from build123d import *

# Parameters (mm, degrees)
SKETCH_1_W          = 117
SKETCH_1_H          = 152
SKETCH_1_R          = 1.525
EXTRUDE_1_DEPTH     = 1
SKETCH_2_R          = 97.5
SKETCH_2_W          = 62.201961009
SKETCH_2_H          = 115
CUT_EXTRUDE_1_DEPTH = 10
SKETCH_3_W          = 20
SKETCH_3_H          = 37.999993186
CUT_EXTRUDE_2_DEPTH = 10
FILLET_1_R          = 2
SKETCH_6_W          = 4
SKETCH_6_H          = 115
EXTRUDE_2_DEPTH     = 1


with BuildPart() as part:
    # 草图1 → 凸台-拉伸1 (new body)
    with BuildSketch(Plane.XY):
        with Locations((38.5, 0)):
            Rectangle(SKETCH_1_W, SKETCH_1_H)
        with Locations((0, 72)):
            Circle(SKETCH_1_R, mode=Mode.SUBTRACT)
        with Locations((0, -72)):
            Circle(SKETCH_1_R, mode=Mode.SUBTRACT)
        with Locations((20, 72)):
            Circle(SKETCH_1_R, mode=Mode.SUBTRACT)
        with Locations((82, 72)):
            Circle(SKETCH_1_R, mode=Mode.SUBTRACT)
        with Locations((82, -72)):
            Circle(SKETCH_1_R, mode=Mode.SUBTRACT)
        with Locations((20, -72)):
            Circle(SKETCH_1_R, mode=Mode.SUBTRACT)
    extrude(amount=EXTRUDE_1_DEPTH)

    # 草图2 → 切除-拉伸1 (cut)
    with BuildSketch(Plane(origin=(0, 0, 0), x_dir=(-1, 0, 0), z_dir=(0, 0, -1))):
        with Locations((101, 0)):
            Circle(SKETCH_2_R)
        with Locations((-65.899019495, 5.300000572)):
            Rectangle(SKETCH_2_W, SKETCH_2_H)
    extrude(amount=-CUT_EXTRUDE_1_DEPTH, mode=Mode.SUBTRACT)

    # 草图3 → 切除-拉伸2 (cut)
    with BuildSketch(Plane(origin=(0, 0, 0), x_dir=(-1, 0, 0), z_dir=(0, 0, -1))):
        with Locations((-30.6, 8.999996593)):
            Rectangle(SKETCH_3_W, SKETCH_3_H)
    extrude(amount=-CUT_EXTRUDE_2_DEPTH, mode=Mode.SUBTRACT)

    # 圆角1
    fillet_1_edges = [part.edges().sort_by_distance(p)[0] for p in [
        (-20, 54.270157545, 0.5),
        (-20, -54.270157545, 0.5),
        (34.798038991, 62.800000572, 0.5),
        (34.798038991, -52.199999428, 0.5),
        (34.798038991, -10, 0.5),
        (34.798038991, 27.999993186, 0.5),
        (20.6, 27.999993186, 0.5),
        (20.6, -10, 0.5),
        (-20, 76, 0.5),
        (97, 76, 0.5),
        (97, -76, 0.5),
        (-20, -76, 0.5),
    ]]
    fillet(fillet_1_edges, radius=FILLET_1_R)

    # 草图6 → 凸台-拉伸2 (add)
    with BuildSketch(Plane.XY.offset(1)):
        with Locations((95, 5.300000572)):
            Rectangle(SKETCH_6_W, SKETCH_6_H)
    extrude(amount=-EXTRUDE_2_DEPTH)


solid = part.part
Design review of the part built by this model. Coordinates are the model's own, in mm. Give positions to 0.01 mm unless a question says otherwise; leave off trailing zeros. Loops run counter-clockwise (first coordinate to the right, second up) from the corner with the lowest first, then second, coordinate; pieces in that order, holes last. Notation, with made-up numbers: M 23,35 L 52,35 A38 ccw 52,74 Z; hole C 59.25,68 d8. An arc over 180 degrees is marked long. Answer as a JSON object with one key per item and string values.
Item 1: Wall thickness on line 1 along Y through (x, z) = (82, 0.3) (3 decimals); line 2 along Y through (x, z) = (20, 0.75) (3 decimals); line 3 along X through (y, z) = (72, 0.6) (3 decimals): over which ranges is each line inside the solid? List them lowest first.
Output values:
{"line 1": "y = -76 to -73.525, -70.475 to -52.2, 62.8 to 70.475, 73.525 to 76", "line 2": "y = -76 to -73.525, -70.475 to 70.475, 73.525 to 76", "line 3": "x = -20 to -1.525, 1.525 to 18.475, 21.525 to 80.475, 83.525 to 97"}
Item 2: Mouldability with a two-part tool opening along X and no side actions: class faces 1 (the face through (-3.503, 0.797, 0.493)), 2 (the face through (12, 1, 0)), 3 (the face through (19.8, -70.49, 0.49)) as pulls with the +X half, pulls with the -X half, needs draft (parallel to the pull), parting line crosses it, or undercut.
Output values:
{"face 1": "pulls with the -X half", "face 2": "needs draft", "face 3": "undercut"}
Item 3: For P1, Ø3.5, axis at x = 0, y = -72, coming from the +Z side; P2, Ø1.8, axis at x = 20, y = -72, coming from the -Z side, all flat-tipped, find the tip position at first contact; note any pin that passes through.
Output values:
{"P1": "stops at z = 1", "P2": "passes through"}
Item 4: We need section C-C (z = 0.6). Count the separate pieces of the cut face and the enclosed holes in it, and give its area (3 significant figures).
Output values:
{"separate pieces": "1", "enclosed holes": "7", "area": "9,290 mm2"}
Item 5: We need section A-A (x = 87.5). State the section outline as (y, z) points, and give its area (3 significant figures).
Output values:
{"outline": "M -76,0 L -52.2,0 L -52.2,1 L -76,1 Z; M 62.8,0 L 76,0 L 76,1 L 62.8,1 Z", "area": "37.0 mm2"}
Item 6: We need section B-B (y = 17.5). State the section outline as (x, z) points.
Output values:
{"outline": "M -5.08,0 L 20.6,0 L 20.6,1 L -5.08,1 Z; M 93,0 L 97,0 L 97,1 L 93,1 Z"}
